Drawing for the job (mm, zero at the part's lowest x, y, z). A direction names the side the tool comes from. Coordinates: 2 decimals unless noted, no trailing zeros. Write each loop counter-clockwise with the first axis right and the second up, starting at its lowest first coordinate (ties: lowest second). Pieces come first, ordered by that corner, then holes. Notation, with made-up numbers: M 65.5,-9 L 82.5,-9 A27 ccw 82.5,13 Z; hole C -6,-9 d9. An arc over 180 degrees is marked long. Put each result on its own line as item: value. Start each with the question number.
Q1. Cut at B-B (y = 1). Write the cut outline in (x, z).
Q2. Drop flat-ended pins along their axis: pin 1 (4 mm diameter, centred on x = 52.5, y = 1.5, fed in from +Z); pin 2 (1 mm diameter, centred on y = 8.5, z = 50, fed in from +X) (1 decimal); pin 3 (3 mm diameter, centred on y = 2.5, z = 47, fed in from +X). Give the stop position or say it passes through.
Q3. Drill centre lines: line 1 along Z through (x, y) = (31.75, 2.5); line 2 along X through (y, z) = (6, 33) (1 decimal); line 3 along Z through (x, y) = (37, 7.75) (1 decimal). Where is each one in solid material? Low to high.
Q4. Cut at D-D (x = 44.5). Write the cut outline in (y, z).
Q5. Pull direction X, two halves, no side cores. Call the marked faces 3, 4 and 5: pulls with the +X half, pulls with the -X half, needs draft (parallel to the pull), parting line crosses it, or undercut.
Q6. Cut at C-C (z = 39). Write the cut outline in (x, y) (1 decimal).
Q7. Cut at A-A (y = 7.25). Give the number of separate pieces and of enclosed holes in the cut face, then the cut area to 3 significant figures.
Q8. Which spindle directions (+Z, -Z, +X, -X, +Y, -Y) get a long thin tool onto all of the face, cutting with end or side? Do the marked faces 1 and 2. Say none if no direction does.
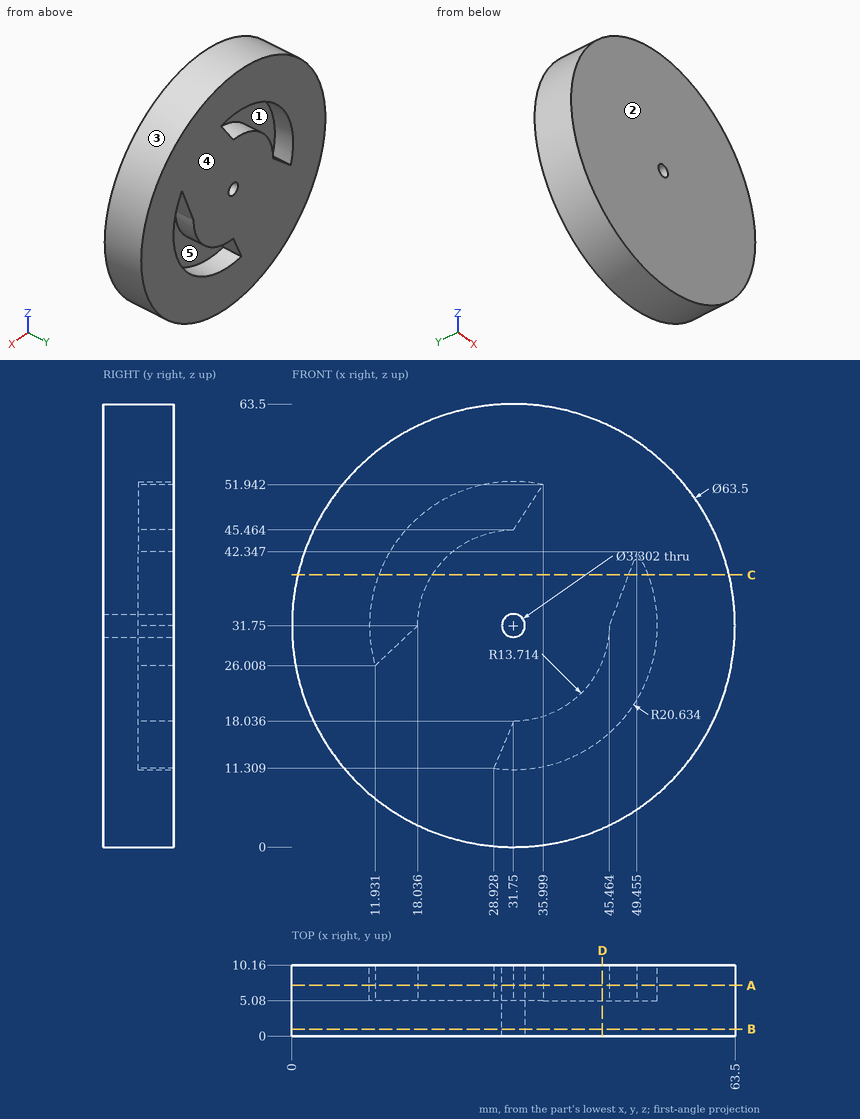
Computed values:
1. outline: C 31.75,31.75 d63.5; hole C 31.75,31.75 d3.3
2. pin 1: z = 57.37
2. pin 2: x = 58.1
2. pin 3: x = 60.37
3. line 1: 0 to 30.1, 33.4 to 63.5
3. line 2: 0 to 11.2, 18.1 to 30.7, 32.8 to 45.9, 52.3 to 63.5
3. line 3: 0.4 to 11.8, 19.1 to 63.1
4. outline: M 0,2.67 L 10.16,2.67 L 10.16,15.53 L 5.08,15.53 L 5.08,26.7 L 10.16,26.7 L 10.16,60.83 L 0,60.83 Z
5. face 3: parting line crosses it
5. face 4: needs draft
5. face 5: undercut
6. outline: M 0.8,0 L 62.7,0 L 62.7,10.2 L 51.1,10.2 L 51.1,5.1 L 48.2,5.1 L 48.2,10.2 L 20.1,10.2 L 20.1,5.1 L 12.4,5.1 L 12.4,10.2 L 0.8,10.2 Z
7. separate pieces: 1
7. enclosed holes: 3
7. area: 2,700 mm2
8. face 1: +Y
8. face 2: +Z, -Z, +X, -X, -Y
